from build123d import *

# Parameters (mm, degrees)
SKETCH_1_W                         = 400
SKETCH_1_H                         = 142
SM_BASE_FLANGE_1_DEPTH             = 0.7
SM_EDGE_FLANGE_1_STRIP_W           = 3.2
SM_EDGE_FLANGE_1_STRIP_H           = 0.7
SM_EDGE_FLANGE_1_STRIP_CUT_DEPTH   = 400
SM_EDGE_FLANGE_1_STRIP_2_W         = 3.2
SM_EDGE_FLANGE_1_STRIP_2_H         = 0.7
SM_EDGE_FLANGE_1_STRIP_CUT_2_DEPTH = 400
SM_EDGE_FLANGE_1_DEPTH             = 400
SM_EDGE_FLANGE_1_BEND_DEPTH        = 400
SKETCH_17_R                        = 3
CUT_EXTRUDE_1_DEPTH                = 10
CUT_EXTRUDE_START                  = -10
SKETCH_18_R                        = 3
CUT_EXTRUDE_2_DEPTH                = 10
SKETCH_19_R                        = 2
CUT_EXTRUDE_3_DEPTH                = 10
SKETCH_20_R                        = 2
CUT_EXTRUDE_4_DEPTH                = 10
SKETCH_21_R                        = 2
CUT_EXTRUDE_5_DEPTH                = 10


# Sheet-metal steps are written as plain solids
with BuildPart() as part:
    # 草图1 → 基体-法兰1 (new body)
    with BuildSketch(Plane(origin=(0, 0, 0), x_dir=(1, 0, 0), z_dir=(0, 1, 0))):
        Rectangle(SKETCH_1_W, SKETCH_1_H)
    extrude(amount=-SM_BASE_FLANGE_1_DEPTH)

    # 边线-法兰1 strip (across the edge) → 边线-法兰1 strip cut (cut)
    with BuildSketch(Plane(origin=(200, 0, -71), x_dir=(0, 0, 1), z_dir=(-1, 0, 0))):
        with Locations((-0.7, -0.35)):
            Rectangle(SM_EDGE_FLANGE_1_STRIP_W, SM_EDGE_FLANGE_1_STRIP_H)
    extrude(amount=SM_EDGE_FLANGE_1_STRIP_CUT_DEPTH, mode=Mode.SUBTRACT)

    # 边线-法兰1 strip 2 (across the edge) → 边线-法兰1 strip cut 2 (cut)
    with BuildSketch(Plane(origin=(-200, 0, 71), x_dir=(0, 0, -1), z_dir=(1, 0, 0))):
        with Locations((-0.7, -0.35)):
            Rectangle(SM_EDGE_FLANGE_1_STRIP_2_W, SM_EDGE_FLANGE_1_STRIP_2_H)
    extrude(amount=SM_EDGE_FLANGE_1_STRIP_CUT_2_DEPTH, mode=Mode.SUBTRACT)

    # 边线-法兰1 section (across the edge) → 边线-法兰1 (add)
    with BuildSketch(Plane(origin=(200, 0, -71), x_dir=(0, 0, 1), z_dir=(-1, 0, 0))):
        with BuildLine():
            Line((0, 0.2), (0, 14.3))
            Line((0, 14.3), (0.7, 14.3))
            Line((0.7, 14.3), (0.7, 0.2))
            ThreePointArc((0.7, 0.2), (0.758578644, 0.058578644), (0.9, 0))
            Line((0.9, 0), (0.9, -0.7))
            ThreePointArc((0.9, -0.7), (0.263603897, -0.436396103), (0, 0.2))
        make_face()
    extrude(amount=SM_EDGE_FLANGE_1_DEPTH)

    # 边线-法兰1 section 2 (across the edge) → 边线-法兰1 bend (add)
    with BuildSketch(Plane(origin=(-200, 0, 71), x_dir=(0, 0, -1), z_dir=(1, 0, 0))):
        with BuildLine():
            Line((0, 0.2), (0, 14.3))
            Line((0, 14.3), (0.7, 14.3))
            Line((0.7, 14.3), (0.7, 0.2))
            ThreePointArc((0.7, 0.2), (0.758578644, 0.058578644), (0.9, 0))
            Line((0.9, 0), (0.9, -0.7))
            ThreePointArc((0.9, -0.7), (0.263603897, -0.436396103), (0, 0.2))
        make_face()
    extrude(amount=SM_EDGE_FLANGE_1_BEND_DEPTH)

    # 草图17 → 切除-拉伸1 (cut)
    with BuildSketch(Plane(origin=(0, 0, -71), x_dir=(-1, 0, 0), z_dir=(0, 0, -1))):
        with Locations(Location((-194.5, 8.8, 0), (0, 0, 90))):
            Circle(SKETCH_17_R)
        with Locations(Location((0, 8.8, 0), (0, 0, 90))):
            Circle(SKETCH_17_R)
        with Locations(Location((194.5, 8.8, 0), (0, 0, 270))):
            Circle(SKETCH_17_R)
    extrude(amount=-CUT_EXTRUDE_1_DEPTH, mode=Mode.SUBTRACT)

    # 草图18 → 切除-拉伸2 (cut)
    with BuildSketch(Plane.XY.offset(71).offset(CUT_EXTRUDE_START)):
        with Locations(Location((-194.5, 8.8, 0), (0, 0, 270))):
            Circle(SKETCH_18_R)
        with Locations(Location((0, 8.8, 0), (0, 0, 90))):
            Circle(SKETCH_18_R)
        with Locations(Location((194.5, 8.8, 0), (0, 0, 90))):
            Circle(SKETCH_18_R)
    extrude(amount=CUT_EXTRUDE_2_DEPTH, mode=Mode.SUBTRACT)

    # 草图19 → 切除-拉伸3 (cut)
    with BuildSketch(Plane(origin=(0, 0, -71), x_dir=(-1, 0, 0), z_dir=(0, 0, -1))):
        with Locations(Location((-170, 8.8, 0), (0, 0, 90))):
            Circle(SKETCH_19_R)
        with Locations(Location((170, 8.8, 0), (0, 0, 270))):
            Circle(SKETCH_19_R)
    extrude(amount=-CUT_EXTRUDE_3_DEPTH, mode=Mode.SUBTRACT)

    # 草图20 → 切除-拉伸4 (cut)
    with BuildSketch(Plane.XY.offset(71).offset(CUT_EXTRUDE_START)):
        with Locations(Location((-170, 8.8, 0), (0, 0, 270))):
            Circle(SKETCH_20_R)
        with Locations(Location((170, 8.8, 0), (0, 0, 90))):
            Circle(SKETCH_20_R)
    extrude(amount=CUT_EXTRUDE_4_DEPTH, mode=Mode.SUBTRACT)

    # 草图21 → 切除-拉伸5 (cut)
    with BuildSketch(Plane(origin=(0, 0, 0), x_dir=(1, 0, 0), z_dir=(0, 1, 0))):
        with Locations(Location((-195, 15, 0), (0, 0, 270))):
            Circle(SKETCH_21_R)
        with Locations(Location((-195, -15, 0), (0, 0, 90))):
            Circle(SKETCH_21_R)
    extrude(amount=-CUT_EXTRUDE_5_DEPTH, mode=Mode.SUBTRACT)


solid = part.part
Build history of the part. All positions in model axes, mm. A direction names the side the tool comes from. Round coordinates to 2 decimals unless told otherwise and drop trailing zeros. Loops run counter-clockwise (first coordinate to the right, second up) from the corner with the lowest first, then second, coordinate; pieces in that order, holes last. Notation, with made-up numbers: (-26, 8.25) -> (6, 8.25) arc R29 cw to (6, 43.25) -> close; hole circle Ø1 at (77, 64.5). An arc over 180 degrees is marked (long way). One line per item, written item: value. Start each with the question number.
Q1. Probe line 1 along X through (y, z) = (8.8, 70.6); line 2 along Z through (x, y) = (32.5, 7); line 3 along Z through (x, y) = (-195, -0.3). List the from-to ranges inside material, lowest first.
Q2. Two-plate mould, pull along Z, no slides. Class faces 3 (the face through (-3, -0.7, -1)), 4 (the face through (3, 7, -71)), 5 (the face through (-3, 7, 71)), 6 (the face through (-3, 7, 70.3)): released by +Z, released by -Z, zero draft, split by the parting line, or undercut.
Q3. Drop flat-ended pins along their axis: pin 1 Ø4.5 at (x, z) = (-195, -15) entering from +Y; pin 2 Ø2.5 at (x, y) = (170, 8.8) entering from +Z. Give the stop position or say it passes through.
Q4. Cut at B-B on x = 69.5. List the corners of the cut face in (y, z).
Q5. Cut at A-A on y = 3. List the corners of the cut face in (x, z).
Q6. 3-axis set-ups, long thin cutter, end or side, ignore diameter. For faces 1 (the face through (200, -0.4, -0.3)), 2 (the face through (3, 7, -70.3)): which of +Z, -Z, +X, -X, +Y, -Y reach the whole face in a straight line?
Q7. Cut at C-C on z = -53. List the corners of the cut face in (x, y).
Computed:
1. line 1: -200 to -197.5, -191.5 to -172, -168 to -3, 3 to 168, 172 to 191.5, 197.5 to 200
1. line 2: -71 to -70.3, 70.3 to 71
1. line 3: -70.85 to -17, -13 to 13, 17 to 70.85
2. face 3: zero draft
2. face 4: released by -Z
2. face 5: released by +Z
2. face 6: undercut
3. pin 1: y = 0
3. pin 2: through
4. outline: (-0.7, -70.1) arc R0.9 ccw to (0.2, -71) -> (14.3, -71) -> (14.3, -70.3) -> (0.2, -70.3) arc R0.2 cw to (0, -70.1) -> (0, 70.1) arc R0.2 cw to (0.2, 70.3) -> (14.3, 70.3) -> (14.3, 71) -> (0.2, 71) arc R0.9 ccw to (-0.7, 70.1) -> close
5. outline: (-200, -71) -> (200, -71) -> (200, -70.3) -> (-200, -70.3) -> close; (-200, 70.3) -> (200, 70.3) -> (200, 71) -> (-200, 71) -> close
6. face 1: +Z, -Z, +X, +Y, -Y
6. face 2: +X, -X, +Y
7. outline: (-200, -0.7) -> (200, -0.7) -> (200, 0) -> (-200, 0) -> close
